Model file for the job. Use its own axes, mm. A direction names the side the tool comes from. Give positions to 0.01 mm unless a question says otherwise; leave off trailing zeros. Write each loop counter-clockwise with the first axis right and the second up, starting at its lowest first coordinate (ties: lowest second). Pieces come first, ordered by that corner, then holes.
Solid Edge part; units mm, degrees
sketch "Sketch1" plane through (0, 0, 0) normal (0, -1, 0) x (1, 0, 0)
  line L0 (-14.5, 8.5) -> (14.5, 8.5)
  line L1 (14.5, 8.5) -> (14.5, -8.5)
  line L2 (14.5, -8.5) -> (-14.5, -8.5)
  line L3 (-14.5, -8.5) -> (-14.5, 8.5)
  dimension "D1" = 14.5
extrude "Protrusion1" add sketch "Sketch1" against normal blind 9.525
hole "Hole_1" at (11.96, 0, -5.155) direction (0, 1, 0) diameter 2.9 end up to next
hole "Hole1" at (-10.27, 0, 5.155) direction (0, 1, 0) diameter 2.9 end up to next
fillet "Round_1" radius 3.175 4 edges at (14.5, 4.7625, -8.5) (-14.5, 4.7625, -8.5) (-14.5, 4.7625, 8.5) (14.5, 4.7625, 8.5)
sketch "Sketch2" plane through (0, 0, 0) normal (0, -1, 0) x (1, 0, 0)
  line L0 (-2.9, 8.5) -> (-2.9, 11.04)
  line L1 (-2.9, 11.04) -> (67, 11.04)
  line L2 (67, 11.04) -> (67, 10.532)
  line L3 (-2.392, 10.532) -> (67, 10.532)
  line L4 (-2.392, 8.5) -> (-2.392, 10.532)
  dimension "D1" = 2.9
  dimension "D2" = 2.9
  dimension "D3" = 2.9
extrude "Protrusion2" add sketch "Sketch2" against normal up to vertex (9.525 mm away) material side at (-2.85, 0, 9.77)
1. Pin check, flat tips, straight feed: P1, Ø2.5, axis at x = 11.96, z = -5.155, coming from the -Y side; P2, Ø3, axis at y = 4, z = -1.5, coming from the +X side; P3, Ø1.5, axis at y = 2, z = 9, coming from the +X side; P4, Ø2, axis at y = 3, z = 10, coming from the -X side. Stop position of each tip, or through.
Calculated:
P1: passes through
P2: stops at x = 14.5
P3: stops at x = 12.56
P4: stops at x = -2.9
2. Slice it at C-C, the plane z = 9.25. Write the cut outline in (x, y) (3 decimals).
Calculated:
outline: (-2.9, 0) - (-2.392, 0) - (-2.392, 9.525) - (-2.9, 9.525) - close
3. Pull direction X, two halves, no side cores. Call faces 1 (the cylindrical face through (-9.834, 4.696, 3.772)), 2 (the cylindrical face through (13.55, 4.83, 7.59)), 3 (the cylindrical face through (13.4, 4.7, -5)), 4 (the flat face through (-7, 5, 8.5)): +X half, -X half, draft (parallel to the pull), parting line (faces both ways), or undercut.
Calculated:
face 1: undercut
face 2: +X half
face 3: undercut
face 4: draft
4. Which spindle directions (+Z, -Z, +X, -X, +Y, -Y) get a long thin tool onto all of the face, cutting with end or side? Do faces 5 (the flat face through (32, 5, 11.04)), 6 (the flat face through (14.5, 5, 0)), 7 (the flat face through (4, 5, 8.5)), 8 (the flat face through (-2.9, 5, 10)). Say none if no direction does.
Calculated:
face 5: +Z, +X, -X, +Y, -Y
face 6: -Z, +X, +Y, -Y
face 7: +X, +Y, -Y
face 8: +Z, -X, +Y, -Y
5. Slice it at B-B, the plane y = 8.25. Write the cut outline in (x, z) (3 decimals).
Calculated:
outline: (-14.5, -5.325) arc R3.175 ccw to (-11.325, -8.5) - (11.325, -8.5) arc R3.175 ccw to (14.5, -5.325) - (14.5, 5.325) arc R3.175 ccw to (11.325, 8.5) - (-2.392, 8.5) - (-2.392, 10.532) - (67, 10.532) - (67, 11.04) - (-2.9, 11.04) - (-2.9, 8.5) - (-11.325, 8.5) arc R3.175 ccw to (-14.5, 5.325) - close; hole circle Ø2.9 at (-10.27, 5.155); hole circle Ø2.9 at (11.96, -5.155)
6. Probe probe 1 along Z at (x, y) = (-10.27, 6.25) (3 decimals); probe 2 along Z at (x, y) = (11.96, 6) (3 decimals); probe 3 along X at (y, z) = (2.25, -1.25). List the from-to ranges inside material, lowest first.
Calculated:
probe 1: z = -8.5 to 3.705, 6.605 to 8.5
probe 2: z = -8.436 to -6.605, -3.705 to 8.436, 10.532 to 11.04
probe 3: x = -14.5 to 14.5
7. Slice it at A-A, the plane x = 6. Write the cut outline in (y, z) (3 decimals).
Calculated:
outline: (0, -8.5) - (9.525, -8.5) - (9.525, 8.5) - (0, 8.5) - close; (0, 10.532) - (9.525, 10.532) - (9.525, 11.04) - (0, 11.04) - close
8. Slice it at D-D, the plane x = -10.27. Write the cut outline in (y, z) (3 decimals).
Calculated:
outline: (0, -8.5) - (9.525, -8.5) - (9.525, 3.705) - (0, 3.705) - close; (0, 6.605) - (9.525, 6.605) - (9.525, 8.5) - (0, 8.5) - close
